```python
from build123d import *

# Parameters (mm, degrees)
F0_R     = 11
F0_R_2   = 5.5
F0_R_3   = 3.95
F0_R_4   = 2.45
F1_DEPTH = 2
F2_DEPTH = 2.6
F3_DEPTH = 8
F4_SIZE  = 0.5
F5_SIZE  = 0.5
F6_SIZE  = 1.5
F7_SIZE  = 1


# Not quite as in the source:
# - a feature names something its author has since deleted; it is built from what else it names


with BuildPart() as f1:
    # F0 (on Top) → F1 (new body)
    with BuildSketch(Plane.XY):
        Circle(F0_R)
        Circle(F0_R_2, mode=Mode.SUBTRACT)
        Circle(F0_R_2)
        Circle(F0_R_3, mode=Mode.SUBTRACT)
        Circle(F0_R_3)
        Circle(F0_R_4, mode=Mode.SUBTRACT)
        Circle(F0_R_4)
    extrude(amount=F1_DEPTH)

    # F0 (on Top) → F2 (join)
    with BuildSketch(Plane.XY):
        Circle(F0_R_2)
        Circle(F0_R_3, mode=Mode.SUBTRACT)
        Circle(F0_R_3)
        Circle(F0_R_4, mode=Mode.SUBTRACT)
        Circle(F0_R_4)
    extrude(amount=F2_DEPTH)

    # F0 (on Top) → F3 (join)
    with BuildSketch(Plane.XY):
        Circle(F0_R_3)
        Circle(F0_R_4, mode=Mode.SUBTRACT)
    extrude(amount=F3_DEPTH)

    # F4
    f4_edges = [f1.edges().sort_by_distance(p)[0] for p in [
        (-2.45, 0, 8),
    ]]
    chamfer(f4_edges, length=F4_SIZE)

    # F5
    f5_edges = [f1.edges().sort_by_distance(p)[0] for p in [
        (-3.95, 0, 8),
    ]]
    chamfer(f5_edges, length=F5_SIZE)

    # F6
    f6_edges = [f1.edges().sort_by_distance(p)[0] for p in [
        (-11, 0, 0),
    ]]
    chamfer(f6_edges, length=F6_SIZE)

    # F7
    f7_edges = [f1.edges().sort_by_distance(p)[0] for p in [
        (-2.45, 0, 2.6),
    ]]
    chamfer(f7_edges, length=F7_SIZE)


solid = f1.part
```
Here's how the part is built. I have some questions about the finished solid (model axes, mm). A direction names the side the tool comes from. Coordinates: 2 decimals unless noted, no trailing zeros. Order: outer loops, then holes, each group sorted by start corner. A loop starts at its lowest first (then second) coordinate and runs counter-clockwise, first axis right, second up. Notation, with made-up numbers: (42, 60.25) - (80, 60.25) arc R15 ccw to (80, 88.25) - close; hole circle Ø4 at (56.25, -27.5). An arc over 180 degrees is marked (long way). One line per question, with ' | ' between items.
(1) If I drill on L1, parallel to X at y = 0, z = 5.4; L2, parallel to Z at x = 5, y = 2, over which ranges is the centre line in solid material (lowest first)?
Report:
L1: x = -3.95 to -2.45, 2.45 to 3.95 | L2: z = 0 to 2.6
(2) If we mould it in two halves opening along Y, with no side actions, what happens to faces 1 (the cylindrical face through (-2.38, -10.74, 1.75)), 2 (the flat face through (-3, 5, 2)), 3 (the flat face through (0, 0, 2.6))? For each: pulls with the +Y half, pulls with the -Y half, needs draft (parallel to the pull), parting line crosses it, or undercut.
Report:
face 1: parting line crosses it | face 2: needs draft | face 3: undercut
(3) Suppose I cut it at A-A on x = 0. List the corners of the cut face in (y, z) for me, and give its area (4 significant figures).
Report:
outline: (-11, 1.5) - (-9.5, 0) - (9.5, 0) - (11, 1.5) - (11, 2) - (5.5, 2) - (5.5, 2.6) - (3.95, 2.6) - (3.95, 7.5) - (3.45, 8) - (2.95, 8) - (2.45, 7.5) - (2.45, 3.6) - (1.45, 2.6) - (-1.45, 2.6) - (-2.45, 3.6) - (-2.45, 7.5) - (-2.95, 8) - (-3.45, 8) - (-3.95, 7.5) - (-3.95, 2.6) - (-5.5, 2.6) - (-5.5, 2) - (-11, 2) - close | area: 65.05 mm2
(4) Will these pins go through, and if not, where does the flat tip stop? pin 1 (1 mm diameter, centred on x = 5.5, y = 2, fed in from -Z); pin 2 (4 mm diameter, centred on x = 0, y = 0, fed in from +Z); pin 3 (1.5 mm diameter, centred on y = -2.5, z = 6, fed in from -X).
Report:
pin 1: stops at z = 0 | pin 2: stops at z = 3.15 | pin 3: stops at x = -3.54
(5) For faces 4 (the cylindrical face through (-1.19, -5.37, 2.3)), 5 (the flat face through (0, 0, 0)), which set-ups out of +Z, -Z, +X, -X, +Y, -Y let a thin tool reach every point of the face, with its end or its side?
Report:
face 4: +Z | face 5: -Z, +X, -X, +Y, -Y
(6) Suppose I cut it at C-C on z = 4. List the corners of the cut face in (x, y) for me, and give its area (3 significant figures).
Report:
outline: circle Ø7.9 at (0, 0); hole circle Ø4.9 at (0, 0) | area: 30.2 mm2
